Autodesk Inventor part; units mm, degrees
ref_plane "YZ Plane" through (0, 0, 0) normal (1, 0, 0) x (0, 1, 0)
ref_plane "XZ Plane" through (0, 0, 0) normal (0, 1, 0) x (-1, 0, 0)
ref_plane "XY Plane" through (0, 0, 0) normal (0, 0, 1) x (1, 0, 0)
sketch "Sketch1" plane through (0, 0, 0) normal (0, 1, 0) x (-1, 0, 0)
  line L0 (90, 60) -> (-90, 60)
  line L1 (-90, 60) -> (-90, -60)
  line L2 (-90, -60) -> (90, -60)
  line L3 (90, -60) -> (90, 60)
  point P0 (0, 0)
  point P1 (0, 60)
  point P2 (90, 0)
  dimension "d0" = 180
  dimension "d1" = 120
extrude "Plate1" add sketch "Sketch1" along normal mid plane 8
sketch "Sketch2" plane through (0, -4, 0) normal (0, -1, 0) x (1, 0, 0)
  line L0 (65, 35) -> (-28.9693, 0.798) construction
  line L1 (-90, -60) -> (-90, 60)
  line L2 (90, 60) -> (90, -60)
  point P0 (0, 0)
  point P1 (-90, 0)
  dimension "d17" = 100
  dimension "d18" = 25
  dimension "d19" = 25
  dimension "d20" = 70
hole "Hole1" at (65, -4, 35) at (-28.9693, -4, 0.798) direction (0, 1, 0) diameter 17 end through all
fillet "Fillet1" radius 2 4 edges at (90, 0, 60) (-90, 0, 60) (90, 0, -60) (-90, 0, -60)
equation "\"d19\" = d18"
equation "\"d8\" = Thickness"
equation "\"d2\" = Thickness"
equation "\"BendRadius\" = Thickness"
equation "\"BendReliefWidth\" = Thickness"
equation "\"BendReliefDepth\" = 0.5 * Thickness"
equation "\"CornerReliefSize\" = 4 * Thickness"
equation "\"MinimumRemnant\" = 2 * Thickness"
equation "\"TransitionRadius\" = BendRadius"
equation "\"JacobiRadiusSize\" = BendRadius"
equation "\"GapSize\" = Thickness"
properties part number "Ухо на стойку_CPY"
Could you check a few things on this model? Use its own coordinates, in mm. Coordinates: 2 decimals unless noted, no trailing zeros. Write each loop counter-clockwise with the first axis right and the second up, starting at its lowest first coordinate (ties: lowest second). Pieces come first, ordered by that corner, then holes. Notation, with made-up numbers: M -7.5,26 L 29.5,26 A20 cw 29.5,45 Z; hole C 1.5,-19.75 d8. An arc over 180 degrees is marked long. One line per question, with ' | ' between items.
1) If we mould it in two halves opening along X, with no side actions, what happens to faces 1 (the face through (-36.137, 0.056, -3.772)), 2 (the face through (1, 0, -60)), 3 (the face through (90, 0, 1))? For each: released by +X, released by -X, zero draft, split by the parting line, or undercut.
Checks:
face 1: undercut | face 2: zero draft | face 3: released by +X
2) Imagine slicing it at A-A, the plane z = 35. Write out the boundary of the cut face in (x, y), and give its area (3 significant figures).
Checks:
outline: M -90,-4 L 56.5,-4 L 56.5,4 L -90,4 Z; M 73.5,-4 L 90,-4 L 90,4 L 73.5,4 Z | area: 1,300 mm²
3) I need wall thicknesses on probe 1 along X at (y, z) = (-0.5, 35); probe 2 along Z at (x, y) = (65, -0.25); probe 3 along Z at (x, y) = (66, -1.25). Which ranges of each line are inside material? Lowest first, please. Write a range as [from, to].
Checks:
probe 1: [-90, 56.5], [73.5, 90] | probe 2: [-60, 26.5], [43.5, 60] | probe 3: [-60, 26.56], [43.44, 60]
4) Imagine slicing it at C-C, the plane y = 0.25. Write out the boundary of the cut face in (x, z).
Checks:
outline: M -90,-58 A2 ccw -88,-60 L 88,-60 A2 ccw 90,-58 L 90,58 A2 ccw 88,60 L -88,60 A2 ccw -90,58 Z; hole C -28.97,0.8 d17; hole C 65,35 d17
5) Imagine slicing it at B-B, the plane x = 65. Write out the boundary of the cut face in (y, z), and give its area (3 significant figures).
Checks:
outline: M -4,-60 L 4,-60 L 4,26.5 L -4,26.5 Z; M -4,43.5 L 4,43.5 L 4,60 L -4,60 Z | area: 824 mm²
